```python
from build123d import *

# Parameters (mm, degrees)
EXTRUDE_1_DEPTH             = 11
CUT_EXTRUDE_1_REACH         = 24
SKETCH_2_R                  = 11.5
HOLE_WIZARD_M4_1_D          = 3.3
HOLE_WIZARD_M4_1_DEPTH      = 10.1
HOLE_WIZARD_M4_1_TIP        = 0.991420021
SKETCH_9_W                  = 51
SKETCH_9_H                  = 32
EXTRUDE_2_DEPTH             = 5
HOLE_WIZARD_3_2_3_2_1_D     = 3.2
HOLE_WIZARD_3_2_3_2_1_DEPTH = 5


with BuildPart() as part:
    # 草图1 → 凸台-拉伸1 (new body, symmetric)
    with BuildSketch(Plane.XY):
        with BuildLine():
            Line((15.5, -15.5), (-15.5, -15.5))
            Line((-15.5, -15.5), (-15.5, 12.63922466))
            ThreePointArc((-15.5, 12.63922466), (-14.142135624, 14.142135624), (-12.63922466, 15.5))
            Line((-12.63922466, 15.5), (12.63922466, 15.5))
            ThreePointArc((12.63922466, 15.5), (14.142135624, 14.142135624), (15.5, 12.63922466))
            Line((15.5, 12.63922466), (15.5, -15.5))
        make_face()
    extrude(amount=EXTRUDE_1_DEPTH, both=True)

    # 草图2 → 切除-拉伸1 (cut, up to next)
    with BuildSketch(Plane.XY.offset(11), mode=Mode.PRIVATE) as cut_extrude_1_sk1:
        Circle(SKETCH_2_R)
    cut_extrude_1_tool1 = extrude(cut_extrude_1_sk1.sketch, amount=-CUT_EXTRUDE_1_REACH, mode=Mode.PRIVATE) & part.part
    add(cut_extrude_1_tool1.solids().sort_by_distance((0, 0, 11))[0], mode=Mode.SUBTRACT)

    # M4 螺纹孔1
    with Locations(Plane.XY.offset(11)):
        with Locations((-11.012100522, 11.012100522), (10.960155108, 10.960155108), (10.960155108, -10.960155108), (-10.960155108, -10.960155108)):
            Hole(HOLE_WIZARD_M4_1_D / 2, depth=HOLE_WIZARD_M4_1_DEPTH)
            with Locations((0, 0, -(HOLE_WIZARD_M4_1_DEPTH + HOLE_WIZARD_M4_1_TIP / 2))):  # 118° drill point
                Cone(0, HOLE_WIZARD_M4_1_D / 2, HOLE_WIZARD_M4_1_TIP, mode=Mode.SUBTRACT)

    # 草图9 → 凸台-拉伸2 (add)
    with BuildSketch(Plane.XZ.offset(15.5)):
        Rectangle(SKETCH_9_W, SKETCH_9_H)
    extrude(amount=EXTRUDE_2_DEPTH)

    # Ø3.2 (3.2) 直径孔1
    with Locations(Plane(origin=(0, -20.5, 0), x_dir=(-1, 0, 0), z_dir=(0, -1, 0))):
        with Locations((20, -10), (-20, -10), (-20, 10), (20, 10)):
            Hole(HOLE_WIZARD_3_2_3_2_1_D / 2, depth=HOLE_WIZARD_3_2_3_2_1_DEPTH)


solid = part.part
```
Work out the finished part from the listing and answer in its coordinate system (mm). A direction names the side the tool comes from. Coordinates: 2 decimals unless noted, no trailing zeros. Write each loop counter-clockwise with the first axis right and the second up, starting at its lowest first coordinate (ties: lowest second). Pieces come first, ordered by that corner, then holes. Notation, with made-up numbers: (62, 3) - (76, 3) arc R30 ccw to (76, 40) - close; hole circle Ø10 at (82, 85.5). An arc over 180 degrees is marked (long way). Answer as a JSON object with one key per item and string values.
Q1. Consider L1, parallel to X at y = -18, z = 10; L2, parallel to Z at x = 20, y = -18.2; L3, parallel to X at y = -16, z = -11. Determine where each line is inside the solid, lowest interval first. Write a range as from..to.
Results list:
{"L1": "x = -25.5..-21.6, -18.4..18.4, 21.6..25.5", "L2": "z = -16..-11.6, -8.4..8.4, 11.6..16", "L3": "x = -25.5..-21.25, -18.75..18.75, 21.25..25.5"}
Q2. Find section D-D (z = 10). Write down the section's boundary in (x, y), plus the area to 3 significant figures.
Results list:
{"outline": "(-25.5, -20.5) - (-21.6, -20.5) - (-21.6, -15.5) - (-25.5, -15.5) - close; (-18.4, -20.5) - (18.4, -20.5) - (18.4, -15.5) - (15.5, -15.5) - (15.5, 12.64) arc R20 ccw to (12.64, 15.5) - (-12.64, 15.5) arc R20 ccw to (-15.5, 12.64) - (-15.5, -15.5) - (-18.4, -15.5) - close; (21.6, -20.5) - (25.5, -20.5) - (25.5, -15.5) - (21.6, -15.5) - close; hole circle Ø3.3 at (-11.01, 11.01); hole circle Ø3.3 at (-10.96, -10.96); hole circle Ø23 at (0, 0); hole circle Ø3.3 at (10.96, -10.96); hole circle Ø3.3 at (10.96, 10.96)", "area": "727 mm^2"}
Q3. Which of the six approach directions +Z, -Z, +X, -X, +Y, -Y give full straight-line access (tool end or side, diameter ignored) to faces 4 (the cylindrical face through (-9.7, 10.01, 5.88)), 5 (the flat face through (15.5, -1, 0)), 6 (the flat face through (-7, 11, -11))?
Results list:
{"face 4": "+Z", "face 5": "+Z, -Z, +X, +Y", "face 6": "-Z, +X, -X, +Y"}
Q4. Find section C-C (x = 0). Write down the section's boundary in (y, z), plus the area to 3 significant figures.
Results list:
{"outline": "(-20.5, -16) - (-15.5, -16) - (-15.5, -11) - (-11.5, -11) - (-11.5, 11) - (-15.5, 11) - (-15.5, 16) - (-20.5, 16) - close; (11.5, -11) - (15.5, -11) - (15.5, 11) - (11.5, 11) - close", "area": "336 mm^2"}
Q5. Given pin 1 Ø5 at (x, y) = (6, 6.5) entering from +Z; pin 2 Ø5.5 at (x, y) = (-10.96, -10.96) entering from -Z; pin 3 Ø4 at (x, z) = (-20, -10) entering from +Y; pin 4 Ø1 at (y, z) = (-7, 2.5) entering from -X, each flat-ended and moving along its own axis, determine where each tip first touches the part or whether it passes through.
Results list:
{"pin 1": "passes through", "pin 2": "stops at z = -11", "pin 3": "stops at y = -15.5", "pin 4": "stops at x = -15.5"}
Q6. Find section B-B (y = 0). Write down the section's boundary in (x, z), plus the area to 3 significant figures.
Results list:
{"outline": "(-15.5, -11) - (-11.5, -11) - (-11.5, 11) - (-15.5, 11) - close; (11.5, -11) - (15.5, -11) - (15.5, 11) - (11.5, 11) - close", "area": "176 mm^2"}
Q7. For a pull along X with two mould halves and no side action, classify faces 1 (the flat face through (-7, 11, 11)), 2 (the flat face through (-25.5, -18, 0)), 3 (the conical face through (-11.3, 11.02, 0.08)) as pulls with the +X half, pulls with the -X half, needs draft (parallel to the pull), parting line crosses it, or undercut.
Results list:
{"face 1": "needs draft", "face 2": "pulls with the -X half", "face 3": "undercut"}
Q8. Find section A-A (z = -6). Write down the section's boundary in (x, y), plus the area to 3 significant figures.
Results list:
{"outline": "(-25.5, -20.5) - (25.5, -20.5) - (25.5, -15.5) - (15.5, -15.5) - (15.5, 12.64) arc R20 ccw to (12.64, 15.5) - (-12.64, 15.5) arc R20 ccw to (-15.5, 12.64) - (-15.5, -15.5) - (-25.5, -15.5) - close; hole circle Ø23 at (0, 0)", "area": "793 mm^2"}
